Autodesk Inventor part; units mm, degrees
ref_plane "YZ Plane" through (0, 0, 0) normal (1, 0, 0) x (0, 1, 0)
ref_plane "XZ Plane" through (0, 0, 0) normal (0, 1, 0) x (-1, 0, 0)
ref_plane "XY Plane" through (0, 0, 0) normal (0, 0, 1) x (1, 0, 0)
sketch "Skizze1" plane through (0, 0, 0) normal (0, 1, 0) x (-1, 0, 0)
  line L0 (28.5, 24.5) -> (-28.5, 24.5)
  line L1 (-33.5, 19.5) -> (-33.5, -19.5)
  line L2 (-28.5, -24.5) -> (28.5, -24.5)
  line L3 (33.5, -19.5) -> (33.5, 19.5)
  arc A0 (28.5, -24.5) -> (33.5, -19.5) centre (28.5, -19.5) ccw
  arc A1 (-33.5, -19.5) -> (-28.5, -24.5) centre (-28.5, -19.5) ccw
  arc A2 (-28.5, 24.5) -> (-33.5, 19.5) centre (-28.5, 19.5) ccw
  arc A3 (33.5, 19.5) -> (28.5, 24.5) centre (28.5, 19.5) ccw
  point P0 (0, 0)
  point P1 (-33.5, -24.5)
  point P2 (-33.5, 24.5)
  point P3 (33.5, -24.5)
  point P4 (-33.5, 0)
  point P5 (0, -24.5)
  dimension "d0" = 67
  dimension "d1" = 49
  dimension "d2" = 5
extrude "Extrusion1" add sketch "Skizze1" along normal blind 2
sketch "Skizze2" plane through (0, 0, 0) normal (1, 0, 0) x (0, 1, 0)
  line L0 (0, -19.5) -> (0, 19.5)
  line L1 (0, 19.5) -> (2, 19.5)
  line L2 (2, -19.5) -> (2, 19.5)
  line L3 (0, -19.5) -> (2, -19.5)
  line L4 (0, -24.5) -> (0, -19.5)
  line L5 (0, -19.5) -> (2, -19.5)
  line L6 (2, -24.5) -> (2, -19.5)
  line L7 (0, -24.5) -> (2, -24.5)
  line L8 (0, 19.5) -> (0, 24.5)
  line L9 (0, 24.5) -> (2, 24.5)
  line L10 (2, 19.5) -> (2, 24.5)
  line L11 (0, 19.5) -> (2, 19.5)
  line L12 (-1.8519, 30.001) -> (19.1551, 0)
  line L13 (19.1551, 0) -> (-1.8519, -30.001)
  line L14 (-0.5098, 30.9407) -> (21.1551, 0)
  line L15 (21.1551, 0) -> (-0.5098, -30.9407)
  arc A0 (-0.5098, 30.9407) -> (-1.8519, 30.001) centre (-1.1808, 30.4709) ccw
  arc A1 (-1.8519, -30.001) -> (-0.5098, -30.9407) centre (-1.1808, -30.4709) ccw
  line L16 (-2, 38.9986) -> (-2, -40.7887) construction
  point P0 (0, 0)
  point P1 (2, 0)
  dimension "d5" = 35
  dimension "d7" = 2
  dimension "d8" = 2
extrude "Extrusion2" add sketch "Skizze2" along normal mid plane 80 contours L13 L12 A0 L14 L15 A1
sketch "Skizze3" plane through (0, 2, 0) normal (0, 1, 0) x (1, 0, 0)
  arc A0 (28.5, -24.5) -> (33.5, -19.5) centre (28.5, -19.5) ccw
  line L0 (-28.5, -24.5) -> (28.5, -24.5)
  arc A1 (-33.5, -19.5) -> (-28.5, -24.5) centre (-28.5, -19.5) ccw
  line L1 (-33.5, 19.5) -> (-33.5, -19.5)
  arc A2 (-28.5, 24.5) -> (-33.5, 19.5) centre (-28.5, 19.5) ccw
  line L2 (28.5, 24.5) -> (-28.5, 24.5)
  arc A3 (33.5, 19.5) -> (28.5, 24.5) centre (28.5, 19.5) ccw
  line L3 (33.5, -19.5) -> (33.5, 19.5)
  arc A4 (-28.5, 24.5) -> (-33.5, 19.5) centre (-28.5, 19.5) ccw
  arc A5 (-33.5, -19.5) -> (-28.5, -24.5) centre (-28.5, -19.5) ccw
  line L4 (-28.5, 24.5) -> (-28.5, -24.5)
  line L5 (28.5, 24.5) -> (-28.5, 24.5)
  line L6 (-28.5, -24.5) -> (28.5, -24.5)
  line L7 (28.5, 24.5) -> (28.5, -24.5)
  point P0 (0, 0)
extrude "Extrusion3" add sketch "Skizze3" along normal up to next contours L7 A3 L3 A0 | A1 L1 A2 L4
sketch "Skizze4" plane through (0, 0, 0) normal (0, -1, 0) x (1, 0, 0)
  arc A0 (33.5, 19.5) -> (28.5, 24.5) centre (28.5, 19.5) ccw
  line L0 (-28.5, 24.5) -> (28.5, 24.5)
  arc A1 (-28.5, 24.5) -> (-33.5, 19.5) centre (-28.5, 19.5) ccw
  line L1 (-33.5, -19.5) -> (-33.5, 19.5)
  arc A2 (-33.5, -19.5) -> (-28.5, -24.5) centre (-28.5, -19.5) ccw
  line L2 (28.5, -24.5) -> (-28.5, -24.5)
  arc A3 (28.5, -24.5) -> (33.5, -19.5) centre (28.5, -19.5) ccw
  line L3 (33.5, 19.5) -> (33.5, -19.5)
  line L4 (-26, 17) -> (26, 17)
  line L5 (26, 17) -> (26, -17)
  line L6 (26, -17) -> (-26, -17)
  line L7 (-26, -17) -> (-26, 17)
  line L8 (-28.5, 24.5) -> (28.5, 24.5)
  point P0 (0, 0)
  point P1 (26, 0)
  point P2 (33.5, 0)
  point P3 (0, 17)
  point P4 (0, 24.5)
  dimension "d13" = 34
  dimension "d14" = 52
extrude "Extrusion4" add sketch "Skizze4" along normal blind 2 contours L4 L5 L6 L7
sketch "Skizze5" plane through (0, -2, 0) normal (0, -1, 0) x (1, 0, 0)
  line L0 (-15, -15) -> (15, -15)
  line L1 (15, -15) -> (15, 15)
  line L2 (15, 15) -> (-15, 15)
  line L3 (-15, 15) -> (-15, -15)
  point P0 (0, 0)
  point P1 (15, 0)
  point P2 (0, 15)
  dimension "d17" = 30
extrude "Extrusion5" cut sketch "Skizze5" against normal up to surface (4 mm away)
sketch "Skizze6" plane through (33.5, 0, 19.5) normal (1, 0, 0) x (0, 0, -1)
  line L0 (0, 0) -> (39, 0)
  line L1 (39, 0) -> (39, 5.501)
  line L2 (19.5, 19.1551) -> (39, 5.501)
  line L3 (0, 5.501) -> (19.5, 19.1551)
  line L4 (0, 0) -> (0, 5.501)
  line L5 (19.5, 18.5447) -> (38.5, 5.2408)
  line L6 (38.5, 5.2408) -> (38.5, 0.5)
  line L7 (38.5, 0.5) -> (0.5, 0.5)
  line L8 (0.5, 0.5) -> (0.5, 5.2408)
  line L9 (0.5, 5.2408) -> (19.5, 18.5447)
  line L10 (0.5, 5.2408) -> (0.2132, 5.6503)
  line L11 (0, 5.501) -> (19.5, 19.1551)
  line L12 (38.5, 5.2408) -> (38.7868, 5.6503)
  line L13 (19.5, 19.1551) -> (39, 5.501)
  line L14 (17.5, 17.1443) -> (17.2132, 17.5539)
  line L15 (21.5, 17.1443) -> (21.7868, 17.5539)
  point P0 (19.5, 0)
  dimension "d20" = 0.5
  dimension "d23" = 2
  dimension "d24" = 2
extrude "Extrusion6" cut sketch "Skizze6" against normal through all contours L3 L14 L9 L10 | L12 L5 L15 L2
equation "\"d24\" = d23"
properties part number "small_top"
Here's how the part is built. I have some questions about the finished solid (model axes, mm). A direction names the side the tool comes from. Round coordinates to 2 decimals unless told otherwise and drop trailing zeros. Write each loop counter-clockwise with the first axis right and the second up, starting at its lowest first coordinate (ties: lowest second). Pieces come first, ordered by that corner, then holes.
Q1. Please list where these lines run through material, in increasing order: probe 1 along X at (y, z) = (3.25, -12); probe 2 along Z at (x, y) = (31, 14.5); probe 3 along Z at (x, y) = (32.5, 19.75).
Q2. Will these pins go through, and if not, where does the flat tip stop? P1, Ø5, axis at y = 4, z = -15.5, coming from the +X side; P2, Ø1, axis at x = -8, y = -1.5, coming from the +Z side; P3, Ø6, axis at x = -16, y = 16, coming from the +Z side; P4, Ø10, axis at y = 2.5, z = 8.5, coming from the -X side.
Q3. If we section it at C-C on z = -16: Write out the boundary of the cut face in (x, y), plus the area to 3 significant figures.
Q4. If we section it at D-D on z = 21: Write out the boundary of the cut face in (x, y).
Q5. Which directions (+Z, -Z, +X, -X, +Y, -Y) give clear straight access to the entire face, cutting with the end or side of a thin tool? Please do faces 1 (the flat face through (0, -1, -17)), 2 (the flat face through (0, 2, 17)), 3 (the flat face through (33.5, 7, 0)), 4 (the flat face through (-30.965, 11.276, -10.381)), 5 (the flat face through (0, 0, -15)).
Q6. If we section it at A-A on x = -27: Write out the boundary of the cut face in (y, z), plus the area to 3 significant figures.
Q7. If we section it at B-B on y = 11: Write out the boundary of the cut face in (x, z).
Q8. If we mould it in two halves opening along Y, with no side actions, what happens to faces 6 (the flat face through (-28.5, 9, 0)), 7 (the flat face through (-0.56, 10.474, -15.254)), 8 (the flat face through (-40, 16.4, -4.5))? For each: +Y half, -Y half, draft (parallel to the pull), parting line (faces both ways), or undercut.
Answer below:
1. probe 1: x = -33.5 to -28.5, 28.5 to 33.5
1. probe 2: z = -9.5 to -6.65, -5.78 to 5.78, 6.65 to 9.5
1. probe 3: z = -2.01 to 2.01
2. P1: stops at x = 33.5
2. P2: stops at z = 31.29
2. P3: stops at z = 11.65
2. P4: stops at x = -33.5
3. outline: (-40, 7.95) - (-28.5, 7.95) - (40, 7.95) - (40, 9.95) - (-40, 9.95) - close; (-33.5, 0) - (-26, 0) - (-26, -2) - (26, -2) - (26, 0) - (33.5, 0) - (33.5, 7.34) - (28.5, 7.34) - (28.5, 2) - (-28.5, 2) - (-28.5, 7.34) - (-33.5, 7.34) - close
3. area: 451 mm2
4. outline: (-40, 4.45) - (-33.27, 4.45) - (-33.27, 0) - (33.27, 0) - (33.27, 4.45) - (40, 4.45) - (40, 6.45) - (-40, 6.45) - close; hole (-28.5, 2) - (28.5, 2) - (28.5, 4.45) - (-28.5, 4.45) - close
5. face 1: +X, -X, -Y
5. face 2: none
5. face 3: +X, -Y
5. face 4: +X, -X
5. face 5: -Y
6. outline: (-1.85, -30) arc R0.82 ccw to (-0.51, -30.94) - (21.16, 0) - (-0.51, 30.94) arc R0.82 ccw to (-1.85, 30) - (2, 24.5) - (0, 24.5) - (0, -24.5) - (2, -24.5) - close; hole (2, -24.5) - (19.16, 0) - (2, 24.5) - close
6. area: 222 mm2
7. outline: (-40, -14.5) - (40, -14.5) - (40, -11.65) - (-28.5, -11.65) - (-40, -11.65) - close; (-40, 11.65) - (40, 11.65) - (40, 14.5) - (-40, 14.5) - close; (-33.5, -10.77) - (-28.5, -10.77) - (-28.5, 10.77) - (-33.5, 10.77) - close; (28.5, -10.77) - (33.5, -10.77) - (33.5, 10.77) - (28.5, 10.77) - close
8. face 6: undercut
8. face 7: +Y half
8. face 8: draft
